Part model, mm, in its own coordinate system. Give positions to 0.01 mm unless a question says otherwise; leave off trailing zeros. Write each loop counter-clockwise with the first axis right and the second up, starting at its lowest first coordinate (ties: lowest second). Pieces come first, ordered by that corner, then holes. Notation, with made-up numbers: (55.25, -1.5) - (69.25, -1.5) arc R19 ccw to (69.25, 33.5) - close; hole circle Ø1 at (75.5, -29). An arc over 180 degrees is marked (long way). Answer in a Markdown table with one row per item. Add a question column.
1. Probe line 1 along X through (y, z) = (-1, -20); line 2 along Z through (x, y) = (28.8, -0.45); line 3 along Z through (x, y) = (422.8, -0.8). List the from-to ranges inside material, lowest first.
2. Drop a flat-ended pin along its axis: pin 1 Ø10 at (x, z) = (229, -26) entering from +Y. Give the stop position or say it passes through.
3. Band-saw the part on A-A on z = -23. Write the cut outline in (x, y).
4. Band-saw the part on B-B on x = 170. Write the cut outline in (y, z).
5. Band-saw the part on C-C on y = -0.8. State how many separate pieces and enclosed holes the cut face has, plus the area to 3 significant figures.
```python
from build123d import *

# Parameters (mm, degrees)
SKETCH_W            = 482.6
SKETCH_H            = 44
PAD_DEPTH           = 2
POCKET_DEPTH        = 2.001
SKETCH002_R         = 2.75
HOLE_DEPTH          = 2.001
SKETCH003_R         = 1.7
HOLE001_DEPTH       = 2.001
SKETCH004_W         = 170
SKETCH004_H         = 27
POCKET001_DEPTH     = 2.001
LINEARPATTERN_COUNT = 2
LINEARPATTERN_PITCH = 203
SKETCH005_R         = 3.25
POCKET002_DEPTH     = 2.001
SKETCH006_W         = 9
SKETCH006_H         = 24
POCKET003_DEPTH     = 2.001
FILLET_R            = 1
FILLET001_R         = 2


with BuildPart() as part:
    # Sketch → Pad (new body)
    with BuildSketch(Plane.XZ):
        with Locations((241.3, -22)):
            Rectangle(SKETCH_W, SKETCH_H)
    extrude(amount=PAD_DEPTH)

    # Sketch001 (on Face6 of Pad) → Pocket (cut, through all)
    with BuildSketch(Plane.XZ.offset(2)):
        with BuildLine():
            ThreePointArc((471.35, -34.375), (467.85, -37.875), (471.35, -41.375))
            Line((471.35, -41.375), (476.35, -41.375))
            ThreePointArc((476.35, -41.375), (479.85, -37.875), (476.35, -34.375))
            Line((471.35, -34.375), (476.35, -34.375))
        make_face()
        with BuildLine():
            ThreePointArc((6.25, -34.375), (2.75, -37.875), (6.25, -41.375))
            Line((6.25, -41.375), (11.25, -41.375))
            ThreePointArc((11.25, -41.375), (14.75, -37.875), (11.25, -34.375))
            Line((6.25, -34.375), (11.25, -34.375))
        make_face()
        with BuildLine():
            ThreePointArc((471.35, -2.625), (467.85, -6.125), (471.35, -9.625))
            Line((471.35, -9.625), (476.35, -9.625))
            ThreePointArc((476.35, -9.625), (479.85, -6.125), (476.35, -2.625))
            Line((471.35, -2.625), (476.35, -2.625))
        make_face()
        with BuildLine():
            ThreePointArc((6.25, -2.625), (2.75, -6.125), (6.25, -9.625))
            Line((6.25, -9.625), (11.25, -9.625))
            ThreePointArc((11.25, -9.625), (14.75, -6.125), (11.25, -2.625))
            Line((6.25, -2.625), (11.25, -2.625))
        make_face()
    extrude(amount=-POCKET_DEPTH, mode=Mode.SUBTRACT)

    # Sketch002 (on Face5 of Pocket) → Hole (cut, through all)
    with BuildSketch(Plane.XZ.offset(2)):
        with Locations((28.8, -12)):
            Circle(SKETCH002_R)
        with Locations((28.8, -32)):
            Circle(SKETCH002_R)
        with Locations((453.8, -12)):
            Circle(SKETCH002_R)
        with Locations((453.8, -32)):
            Circle(SKETCH002_R)
    extrude(amount=-HOLE_DEPTH, mode=Mode.SUBTRACT)

    # Sketch003 (on Face5 of Hole) → Hole001 (cut, through all)
    with BuildSketch(Plane.XZ.offset(2)):
        with Locations((438.3, -7.25)):
            Circle(SKETCH003_R)
        with Locations((247.3, -7.25)):
            Circle(SKETCH003_R)
        with Locations((235.3, -7.25)):
            Circle(SKETCH003_R)
        with Locations((44.3, -7.25)):
            Circle(SKETCH003_R)
    extrude(amount=-HOLE001_DEPTH, mode=Mode.SUBTRACT)

    # Sketch004 (on Face5 of Hole001) → Pocket001 (cut, through all)
    with BuildSketch(Plane.XZ.offset(2)):
        with Locations((127.8, -25.25)):
            Rectangle(SKETCH004_W, SKETCH004_H)
    pocket001 = extrude(amount=-POCKET001_DEPTH, mode=Mode.SUBTRACT)

    # LinearPattern: Pocket001 ×2
    with Locations(*[(i * LINEARPATTERN_PITCH, 0, 0) for i in range(1, LINEARPATTERN_COUNT)]):
        add(pocket001, mode=Mode.SUBTRACT)

    # Sketch005 (on Face5 of LinearPattern) → Pocket002 (cut, through all)
    with BuildSketch(Plane.XZ.offset(2)):
        with Locations((422.8, -13.25)):
            Circle(SKETCH005_R)
        with Locations((422.8, -30.25)):
            Circle(SKETCH005_R)
    extrude(amount=-POCKET002_DEPTH, mode=Mode.SUBTRACT)

    # Sketch006 (on Face5 of Pocket002) → Pocket003 (cut, through all)
    with BuildSketch(Plane.XZ.offset(2)):
        with Locations((434.7, -25.25)):
            Rectangle(SKETCH006_W, SKETCH006_H)
    extrude(amount=-POCKET003_DEPTH, mode=Mode.SUBTRACT)

    # Fillet
    fillet_edges = [part.edges().sort_by_distance(p)[0] for p in [
        (439.2, -1, -13.25),
        (430.2, -1, -13.25),
        (430.2, -1, -37.25),
        (439.2, -1, -37.25),
        (415.8, -1, -11.75),
        (415.8, -1, -38.75),
        (245.8, -1, -11.75),
        (245.8, -1, -38.75),
        (42.8, -1, -38.75),
        (42.8, -1, -11.75),
        (212.8, -1, -11.75),
        (212.8, -1, -38.75),
    ]]
    fillet(fillet_edges, radius=FILLET_R)

    # Fillet001
    fillet001_edges = [part.edges().sort_by_distance(p)[0] for p in [
        (482.6, -1, -44),
        (482.6, -1, 0),
        (0, -1, -44),
        (0, -1, 0),
    ]]
    fillet(fillet001_edges, radius=FILLET001_R)


solid = part.part
```
Values:
| question | item | result |
|---|---|---|
| 1 | line 1 | x = 0 to 42.8, 212.8 to 245.8, 415.8 to 430.2, 439.2 to 482.6 |
| 1 | line 2 | z = -44 to -34.75, -29.25 to -14.75, -9.25 to 0 |
| 1 | line 3 | z = -44 to -33.5, -27 to -16.5, -10 to 0 |
| 2 | pin 1 | stops at y = 0 |
| 3 | outline | (0, -2) - (42.8, -2) - (42.8, 0) - (0, 0) - close; (212.8, -2) - (245.8, -2) - (245.8, 0) - (212.8, 0) - close; (415.8, -2) - (430.2, -2) - (430.2, 0) - (415.8, 0) - close; (439.2, -2) - (482.6, -2) - (482.6, 0) - (439.2, 0) - close |
| 4 | outline | (-2, -44) - (0, -44) - (0, -38.75) - (-2, -38.75) - close; (-2, -11.75) - (0, -11.75) - (0, 0) - (-2, 0) - close |
| 5 | separate pieces | 1 |
| 5 | enclosed holes | 17 |
| 5 | area | 11,300 mm² |
